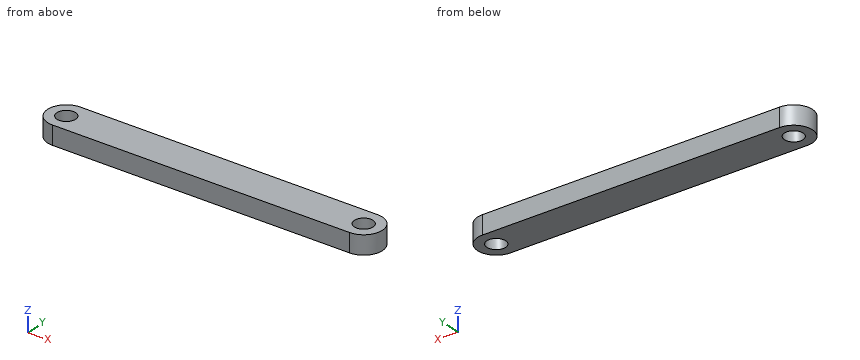
Autodesk Inventor part; units mm, degrees
ref_plane "YZ Plane" through (0, 0, 0) normal (1, 0, 0) x (0, 1, 0)
ref_plane "XZ Plane" through (0, 0, 0) normal (0, 1, 0) x (-1, 0, 0)
ref_plane "XY Plane" through (0, 0, 0) normal (0, 0, 1) x (1, 0, 0)
sketch "Sketch1" plane through (0, 0, 0) normal (0, 0, 1) x (1, 0, 0)
  line L0 (0, 0) -> (-50.8, 0)
  line L1 (-50.8, 0) -> (-50.8, 6.35)
  line L2 (-50.8, 6.35) -> (0, 6.35)
  line L3 (0, 6.35) -> (0, 0)
  arc A0 (-50.8, 6.35) -> (-50.8, 0) centre (-50.8, 3.175) ccw
  arc A1 (0, 0) -> (0, 6.35) centre (0, 3.175) ccw
  circle A2 centre (-50.8, 3.175) radius 1.5875
  circle A3 centre (0, 3.175) radius 1.5875
  dimension "d0" = 50.8
  dimension "d1" = 6.35
  dimension "d2" = 3.175
  dimension "d3" = 3.175
  dimension "d4" = 3.175
extrude "Extrusion1" add sketch "Sketch1" along normal blind 3.175
extrude "Extrusion2" cut sketch "Sketch1" along normal blind 3.175 contours A3 L3 | L3 A3 | A2 L1 | L1 A2
For this review, take the finished solid that the model builds, in its own axes (mm). Give positions to 0.01 mm unless a question says otherwise; leave off trailing zeros. Loops run counter-clockwise (first coordinate to the right, second up) from the corner with the lowest first, then second, coordinate; pieces in that order, holes last.
Item 1: Take a section at D-D, the plane y = 0.5. State the section outline as (x, z) points (3 decimals).
Item 2: For line 1 along X through (y, z) = (2, 3); line 2 along X through (y, z) = (2.5, 0.4); line 3 along Y through (x, z) = (0, 2.2), list the stretches that pass through material, from the lowest coordinate up.
Item 3: Insertion check: pin 1 (1 mm diameter, centred on y = 2.5, z = 1.5, fed in from +X). The pin has a flat end and moves straight along its axis. Give the tip position at first contact, or say it passes through.
Item 4: Take a section at B-B, the plane z = 1.25. Give the number of separate pieces and of enclosed holes in the cut face, and give its area (3 significant figures).
Item 5: Take a section at A-A, the plane y = 4. State the section outline as (x, z) points (3 decimals), and give its area (3 significant figures).
Item 6: Take a section at C-C, the plane x = -1. State the section outline as (y, z) points (3 decimals).
Calculated:
1. outline: (-52.51, 0) - (1.71, 0) - (1.71, 3.175) - (-52.51, 3.175) - close
2. line 1: x = -53.75 to -51.87, -49.73 to -1.07, 1.07 to 2.95
2. line 2: x = -53.9 to -52.24, -49.36 to -1.44, 1.44 to 3.1
2. line 3: y = 0 to 1.59, 4.76 to 6.35
3. pin 1: stops at x = 3.17
4. separate pieces: 1
4. enclosed holes: 2
4. area: 338 mm2
5. outline: (-53.866, 0) - (-52.156, 0) - (-52.156, 3.175) - (-53.866, 3.175) - close; (-49.444, 0) - (-1.356, 0) - (-1.356, 3.175) - (-49.444, 3.175) - close; (1.356, 0) - (3.066, 0) - (3.066, 3.175) - (1.356, 3.175) - close
5. area: 164 mm2
6. outline: (0, 0) - (1.942, 0) - (1.942, 3.175) - (0, 3.175) - close; (4.408, 0) - (6.35, 0) - (6.35, 3.175) - (4.408, 3.175) - close
